The model under review builds one solid part; all positions refer to its coordinate system, in mm. A direction names the side the tool comes from. Round coordinates to 2 decimals unless told otherwise and drop trailing zeros. Loops run counter-clockwise (first coordinate to the right, second up) from the corner with the lowest first, then second, coordinate; pieces in that order, holes last. Notation, with made-up numbers: (68.25, 15) -> (92.25, 15) arc R14 ccw to (92.25, 38) -> close; hole circle Ø8 at (67.25, 30.5). An arc over 180 degrees is marked (long way). Write each question's results on one line, items separated by ' | '. Start each with the question number.
Item 1: Mouldability with a two-part tool opening along X and no side actions: class faces 4 (the flat face through (-3, 6, 3)), 5 (the flat face through (-1, 0, 2)), 6 (the cylindrical face through (0.78, 5.027, 2.958)) as pulls with the +X half, pulls with the -X half, needs draft (parallel to the pull), parting line crosses it, or undercut.
Item 2: We need section C-C (z = 5.45). Give the boundary of the cut face in (x, y), and give its area (3 significant figures).
Item 3: For L1, parallel to Z at x = -3, y = 3; L2, parallel to X at y = 10.25, z = 2.9; L3, parallel to Y at x = 3.75, z = 4.15, list the stretches that pass through material, from the lowest coordinate up. Write a range as from..to.
Item 4: Tool access review of faces 1 (the flat face through (4, 6, 3)), 2 (the flat face through (-0.686, 9, 3)), 3 (the flat face through (5.314, 10, 1)): name each direction out of +Z, -Z, +X, -X, +Y, -Y from which nothing blocks a thin tool from reaching the whole face with its end or side.
Item 5: Clearance check with flat-ended pins moving along their axes: pin 1 Ø0.8 at (x, z) = (4.5, 4) entering from -Y; pin 2 Ø3.5 at (y, z) = (1, 4) entering from +X; pin 3 Ø1.2 at (y, z) = (9.5, 3.5) entering from +X. State where each tip first meets the part, or that it passes through.
Item 6: We need section B-B (y = 1.5). Give the boundary of the cut face in (x, z), and give its area (3 significant figures).
Item 7: We need section D-D (x = -3). Give the boundary of the cut face in (y, z), and give its area (3 significant figures).
Item 8: We need section A-A (x = 3.5). Give the boundary of the cut face in (y, z).
from build123d import *

# Parameters (mm, degrees)
BOSS_EXTRUDE2_DEPTH = 6
CUT_EXTRUDE6_DEPTH  = 6
CUT_EXTRUDE7_DEPTH  = 6


with BuildPart() as part:
    # Sketch1 → Boss-Extrude2 (new body)
    with BuildSketch(Plane.XY):
        with BuildLine():
            Line((-4.773172478, 12), (5.313782991, 12))
            Line((5.313782991, 12), (5.313782991, 6))
            Line((5.313782991, 6), (2.656891496, 6))
            ThreePointArc((2.656891496, 6), (0.759711241, 5.003688625), (0, 3))
            Line((0, 3), (0, 0))
            Line((0, 0), (-6, 0))
            Line((-6, 0), (-6, 10.773172478))
            ThreePointArc((-6, 10.773172478), (-5.640670538, 11.640670538), (-4.773172478, 12))
        make_face()
    extrude(amount=BOSS_EXTRUDE2_DEPTH)

    # Sketch5 → Cut-Extrude6 (cut)
    with BuildSketch(Plane(origin=(5.313782991, 0, 0), x_dir=(0, 0, -1), z_dir=(1, 0, 0))):
        with BuildLine():
            ThreePointArc((-1.585786438, 10.414213562), (-4.414213562, 10.414213562), (-4.414213562, 7.585786438))
            Line((-4.414213562, 7.585786438), (-1.585786438, 10.414213562))
        make_face()
        with BuildLine():
            Line((-1.585786438, 10.414213562), (-4.414213562, 7.585786438))
            ThreePointArc((-4.414213562, 7.585786438), (-2.234633135, 7.152240935), (-1, 9))
            ThreePointArc((-1, 9), (-1.152240935, 9.765366865), (-1.585786438, 10.414213562))
        make_face()
    extrude(amount=-CUT_EXTRUDE6_DEPTH, mode=Mode.SUBTRACT)

    # Sketch6 → Cut-Extrude7 (cut)
    with BuildSketch(Plane.XZ):
        with BuildLine():
            ThreePointArc((-1.585786438, 4.414213562), (-4.414213562, 4.414213562), (-4.414213562, 1.585786438))
            Line((-4.414213562, 1.585786438), (-1.585786438, 4.414213562))
        make_face()
        with BuildLine():
            Line((-1.585786438, 4.414213562), (-4.414213562, 1.585786438))
            ThreePointArc((-4.414213562, 1.585786438), (-2.234633135, 1.152240935), (-1, 3))
            ThreePointArc((-1, 3), (-1.152240935, 3.765366865), (-1.585786438, 4.414213562))
        make_face()
    extrude(amount=-CUT_EXTRUDE7_DEPTH, mode=Mode.SUBTRACT)


solid = part.part
Here are the results:
1) face 4: undercut | face 5: needs draft | face 6: pulls with the +X half
2) outline: (-6, 0) -> (0, 0) -> (0, 3) arc R3.02 cw to (2.66, 6) -> (5.31, 6) -> (5.31, 12) -> (-4.77, 12) arc R1.23 ccw to (-6, 10.77) -> close | area: 105 mm2
3) L1: z = 0..1, 5..6 | L2: x = -6..-0.69 | L3: y = 6..7.36, 10.64..12
4) face 1: +Z, -Z, +X, -Y | face 2: +X | face 3: +Z, -Z, +X, +Y, -Y
5) pin 1: stops at y = 6 | pin 2: stops at x = 0 | pin 3: stops at x = -0.69
6) outline: (-6, 0) -> (0, 0) -> (0, 6) -> (-6, 6) -> close; hole circle Ø4 at (-3, 3) | area: 23.4 mm2
7) outline: (0, 0) -> (12, 0) -> (12, 6) -> (0, 6) -> (0, 5) -> (6, 5) -> (6, 1) -> (0, 1) -> close | area: 48.0 mm2
8) outline: (6, 0) -> (12, 0) -> (12, 6) -> (6, 6) -> close; hole circle Ø4 at (9, 3)
